Autodesk Inventor part; units mm, degrees
ref_plane "YZ Plane" through (0, 0, 0) normal (1, 0, 0) x (0, 1, 0)
ref_plane "XZ Plane" through (0, 0, 0) normal (0, 1, 0) x (-1, 0, 0)
ref_plane "XY Plane" through (0, 0, 0) normal (0, 0, 1) x (1, 0, 0)
sketch "Sketch1" plane through (0, 0, 0) normal (0, 1, 0) x (-1, 0, 0)
  line L0 (0, 0) -> (-299.72, 0)
  line L1 (-299.72, 0) -> (-299.72, 222.25)
  line L2 (-299.72, 222.25) -> (0, 222.25)
  line L3 (0, 222.25) -> (0, 0)
  dimension "d0" = 299.72
  dimension "d1" = 222.25
extrude "Extrusion1" add sketch "Sketch1" along normal blind 6.35
sketch "Sketch2" plane through (0, 6.35, 0) normal (0, 1, 0) x (1, 0, 0)
  line L0 (0, 0) -> (0, -222.25)
  line L1 (299.72, -222.25) -> (299.72, 0)
  line L2 (0, -222.25) -> (299.72, -222.25)
  line L3 (299.72, -222.25) -> (299.72, 0)
  line L4 (299.72, 0) -> (0, 0)
  line L5 (0, 0) -> (0, -222.25)
  line L6 (296.545, -219.075) -> (3.175, -219.075)
  line L7 (3.175, -219.075) -> (3.175, -3.175)
  line L8 (3.175, -3.175) -> (296.545, -3.175)
  line L9 (296.545, -3.175) -> (296.545, -219.075)
  point P0 (299.72, -222.25)
  dimension "d4" = 3.175
extrude "Extrusion2" add sketch "Sketch2" along normal blind 76.2
sketch "Sketch3" plane through (0, 6.35, 0) normal (0, 1, 0) x (1, 0, 0)
  line L0 (3.175, -219.075) -> (3.175, -3.175) construction
  line L1 (3.175, -3.175) -> (28.575, -3.175) construction
  line L2 (28.575, -3.175) -> (28.575, -28.575) construction
  line L3 (28.575, -28.575) -> (3.175, -28.575) construction
  line L4 (3.175, -28.575) -> (3.175, -3.175) construction
  line L5 (296.545, -3.175) -> (271.145, -3.175) construction
  line L6 (271.145, -3.175) -> (271.145, -28.575) construction
  line L7 (271.145, -28.575) -> (296.545, -28.575) construction
  line L8 (296.545, -28.575) -> (296.545, -3.175) construction
  line L9 (296.545, -219.075) -> (3.175, -219.075) construction
  line L10 (296.545, -219.075) -> (271.145, -219.075) construction
  line L11 (271.145, -219.075) -> (271.145, -193.675) construction
  line L12 (271.145, -193.675) -> (296.545, -193.675) construction
  line L13 (296.545, -193.675) -> (296.545, -219.075) construction
  line L14 (3.175, -219.075) -> (28.575, -219.075) construction
  line L15 (28.575, -219.075) -> (28.575, -193.675) construction
  line L16 (28.575, -193.675) -> (3.175, -193.675) construction
  line L17 (3.175, -193.675) -> (3.175, -219.075) construction
  line L18 (3.175, -193.675) -> (28.575, -219.075) construction
  line L19 (28.575, -193.675) -> (3.175, -219.075) construction
  line L20 (271.145, -193.675) -> (296.545, -219.075) construction
  line L21 (296.545, -219.075) -> (296.545, -193.675) construction
  line L22 (296.545, -193.675) -> (271.145, -219.075) construction
  line L23 (271.145, -3.175) -> (296.545, -28.575) construction
  line L24 (296.545, -3.175) -> (271.145, -28.575) construction
  line L25 (3.175, -3.175) -> (28.575, -28.575) construction
  line L26 (28.575, -3.175) -> (3.175, -28.575) construction
  circle A0 centre (15.875, -15.875) radius 2.3812
  circle A1 centre (283.845, -15.875) radius 2.3812
  circle A2 centre (283.845, -206.375) radius 2.3812
  circle A3 centre (15.875, -206.375) radius 2.3813
  point P0 (0, 0)
  dimension "d7" = 25.4
  dimension "d8" = 25.4
  dimension "d9" = 25.4
  dimension "d10" = 25.4
  dimension "d11" = 25.4
  dimension "d12" = 25.4
  dimension "d13" = 25.4
  dimension "d14" = 25.4
  dimension "d15" = 4.7625
  dimension "d16" = 4.7625
  dimension "d17" = 4.7625
  dimension "d18" = 4.7625
extrude "Extrusion3" cut sketch "Sketch3" against normal blind 6.35
sketch "Sketch4" plane through (3.175, 6.35, 219.075) normal (1, 0, 0) x (0, 0, -1)
  line L0 (215.9, 0) -> (0, 0) construction
  line L1 (0, 0) -> (25.4, 0) construction
  line L2 (25.4, 0) -> (25.4, 25.4) construction
  line L3 (25.4, 25.4) -> (0, 25.4) construction
  line L4 (0, 25.4) -> (0, 0) construction
  line L5 (215.9, 0) -> (190.5, 0) construction
  line L6 (190.5, 0) -> (190.5, 25.4) construction
  line L7 (190.5, 25.4) -> (215.9, 25.4) construction
  line L8 (215.9, 25.4) -> (215.9, 0) construction
  line L9 (0, 25.4) -> (25.4, 0) construction
  line L10 (25.4, 25.4) -> (0, 0) construction
  line L11 (190.5, 25.4) -> (215.9, 0) construction
  line L12 (215.9, 25.4) -> (190.5, 0) construction
  circle A0 centre (203.2, 12.7) radius 2.3813
  circle A1 centre (12.7, 12.7) radius 2.3813
  point P0 (219.075, -6.35)
  dimension "d21" = 25.4
  dimension "d22" = 25.4
  dimension "d23" = 25.4
  dimension "d24" = 25.4
  dimension "d25" = 4.7625
  dimension "d26" = 4.7625
extrude "Extrusion4" cut sketch "Sketch4" against normal blind 3.175
sketch "Sketch5" plane through (3.175, 6.35, 3.175) normal (0, 0, 1) x (1, 0, 0)
  line L0 (0, 0) -> (0, 76.2) construction
  line L1 (0, 0) -> (25.4, 0) construction
  line L2 (25.4, 0) -> (25.4, 25.4) construction
  line L3 (25.4, 25.4) -> (0, 25.4) construction
  line L4 (0, 25.4) -> (0, 0) construction
  line L5 (293.37, 0) -> (267.97, 0) construction
  line L6 (267.97, 0) -> (267.97, 25.4) construction
  line L7 (267.97, 25.4) -> (293.37, 25.4) construction
  line L8 (293.37, 25.4) -> (293.37, 0) construction
  line L9 (0, 25.4) -> (25.4, 0) construction
  line L10 (293.37, 0) -> (0, 0) construction
  line L11 (25.4, 25.4) -> (0, 0) construction
  line L12 (293.37, 25.4) -> (267.97, 0) construction
  line L13 (293.37, 0) -> (293.37, 76.2) construction
  line L14 (267.97, 25.4) -> (293.37, 0) construction
  circle A0 centre (280.67, 12.7) radius 2.3812
  circle A1 centre (12.7, 12.7) radius 2.3813
  point P0 (-3.175, -6.35)
  dimension "d29" = 25.4
  dimension "d30" = 25.4
  dimension "d31" = 25.4
  dimension "d32" = 25.4
  dimension "d33" = 4.7625
  dimension "d34" = 4.7625
extrude "Extrusion5" cut sketch "Sketch5" against normal blind 3.175
sketch "Sketch6" plane through (296.545, 6.35, 3.175) normal (-1, 0, 0) x (0, 0, 1)
  line L0 (215.9, 0) -> (0, 0) construction
  line L1 (0, 0) -> (25.4, 0) construction
  line L2 (25.4, 0) -> (25.4, 25.4) construction
  line L3 (25.4, 25.4) -> (0, 25.4) construction
  line L4 (0, 25.4) -> (0, 0) construction
  line L5 (215.9, 0) -> (190.5, 0) construction
  line L6 (190.5, 0) -> (190.5, 25.4) construction
  line L7 (190.5, 25.4) -> (215.9, 25.4) construction
  line L8 (215.9, 25.4) -> (215.9, 0) construction
  line L9 (190.5, 0) -> (215.9, 25.4) construction
  line L10 (215.9, 0) -> (215.9, 76.2) construction
  line L11 (190.5, 25.4) -> (215.9, 0) construction
  line L12 (0, 25.4) -> (25.4, 0) construction
  line L13 (25.4, 25.4) -> (0, 0) construction
  circle A0 centre (12.7, 12.7) radius 2.3812
  circle A1 centre (203.2, 12.7) radius 2.3813
  point P0 (-3.175, -6.35)
  dimension "d37" = 25.4
  dimension "d38" = 25.4
  dimension "d39" = 25.4
  dimension "d40" = 25.4
  dimension "d41" = 4.7625
  dimension "d42" = 4.7625
extrude "Extrusion6" cut sketch "Sketch6" against normal blind 3.175
sketch "Sketch7" plane through (296.545, 6.35, 219.075) normal (0, 0, -1) x (-1, 0, 0)
  line L0 (293.37, 0) -> (267.97, 0) construction
  line L1 (267.97, 0) -> (267.97, 25.4) construction
  line L2 (267.97, 25.4) -> (293.37, 25.4) construction
  line L3 (293.37, 25.4) -> (293.37, 0) construction
  line L4 (293.37, 0) -> (0, 0) construction
  line L5 (0, 0) -> (25.4, 0) construction
  line L6 (25.4, 0) -> (25.4, 25.4) construction
  line L7 (25.4, 25.4) -> (0, 25.4) construction
  line L8 (0, 25.4) -> (0, 0) construction
  line L9 (0, 25.4) -> (25.4, 0) construction
  line L10 (25.4, 25.4) -> (0, 0) construction
  line L11 (267.97, 0) -> (293.37, 25.4) construction
  line L12 (267.97, 25.4) -> (293.37, 0) construction
  circle A0 centre (280.67, 12.7) radius 2.3812
  circle A1 centre (12.7, 12.7) radius 2.3813
  point P0 (296.545, -6.35)
  dimension "d45" = 25.4
  dimension "d46" = 25.4
  dimension "d47" = 25.4
  dimension "d48" = 25.4
  dimension "d49" = 4.7625
  dimension "d50" = 4.7625
extrude "Extrusion7" cut sketch "Sketch7" against normal blind 3.175
sketch "Sketch8" plane through (3.175, 6.35, 219.075) normal (1, 0, 0) x (0, 0, -1)
  line L0 (215.9, 0) -> (0, 0) construction
  line L1 (0, 0) -> (107.95, 0) construction
  line L2 (107.95, 0) -> (130.175, 0) construction
  line L3 (107.95, 0) -> (130.175, 0) construction
  line L4 (130.175, 0) -> (85.725, 0) construction
  line L5 (85.725, 0) -> (85.725, 20.6375) construction
  line L6 (85.725, 20.6375) -> (130.175, 20.6375) construction
  line L7 (130.175, 20.6375) -> (130.175, 0) construction
  line L8 (85.725, 0) -> (85.725, 10.3251) construction
  line L9 (130.175, 0) -> (130.175, 10.3251) construction
  line L10 (130.175, 0) -> (140.5001, 0) construction
  line L11 (85.725, 10.3251) -> (87.3125, 10.3251) construction
  line L12 (130.175, 10.3251) -> (128.5875, 10.3251) construction
  line L13 (128.5875, 10.3251) -> (120.65, 10.3251) construction
  line L14 (128.5875, 10.3251) -> (136.525, 10.3251) construction
  line L15 (87.3125, 10.3251) -> (95.25, 10.3251) construction
  line L16 (87.3125, 10.3251) -> (95.25, 10.3251) construction
  circle A0 centre (95.25, 10.3251) radius 7.9375
  circle A1 centre (120.65, 10.3251) radius 7.9375
  dimension "d53" = 107.95
  dimension "d54" = 22.225
  dimension "d55" = 0
  dimension "d56" = 44.45
  dimension "d57" = 20.6375
  dimension "d58" = 10.3251
  dimension "d59" = 10.3251
  dimension "d60" = 90
  dimension "d61" = 1.5875
  dimension "d62" = 1.5875
  dimension "d64" = 7.9375
  dimension "d65" = 180
  dimension "d66" = 7.9375
  dimension "d67" = 0
  dimension "d68" = 15.875
  dimension "d69" = 15.875
extrude "Extrusion8" cut sketch "Sketch8" against normal blind 3.175
properties part number "Lower Chassis_2"
Input: part model. Units: mm. Frame: model coordinates. A direction names the side the tool comes from. Coordinates: 2 decimals unless noted, no trailing zeros. Loops run counter-clockwise (first coordinate to the right, second up) from the corner with the lowest first, then second, coordinate; pieces in that order, holes last. Notation, with made-up numbers: (69, 61) -> (88, 61) arc R15 cw to (88, 67) -> close; hole circle Ø10 at (-20, -15.5). An arc over 180 degrees is marked (long way). Write item = value, one per line. Start each with the question number.
Item 1: Cut plane B-B, the plane x = 162. Return loops of the section in (y, z) (3 decimals).
Item 2: Material intervals for line 1 (Z direction, x = 279.5, y = 38) (3 decimals); line 2 (X direction, y = 52, z = 30.5) (3 decimals); line 3 (Z direction, x = 2, y = 19), sorted ascending.
Item 3: First-contact query: P1, Ø4, axis at x = 15.875, z = 15.875, coming from the -Y side; P2, Ø7.5, axis at x = 283.845, z = 15.875, coming from the +Y side. Flat tips, straight axial feed; report the tip coordinate or a pass-through.
Item 4: Cut plane A-A, the plane y = 67. Return loops of the section in (x, z) (3 decimals), plus the area to 3 significant figures.
Item 5: Reachability of faces 5 (the face through (299.72, 41, 110)), 6 (the face through (152, 44, 219.075)), 7 (the face through (1.61, 13.635, 116.493)) from +Z, -Z, +X, -X, +Y, -Y: full face, straight path, thin tool, end or side. Return the list, or none.
Item 6: Cut plane C-C, the plane z = 148. Return loops of the section in (x, y) (3 decimals), plus the area to 3 significant figures.
Item 7: Mould query, pull axis Z, two halves, no side actions, for faces 1 (the face through (148, 44, 3.175)), 2 (the face through (1.61, 13.635, 91.093)), 3 (the face through (152, 41, 222.25)), 4 (the face through (0, 41, 113)). Classes: pulls with the +Z half, pulls with the -Z half, needs draft (parallel to the pull), parting line crosses it, or undercut.
Ans:
q1.outline = (0, 0) -> (82.55, 0) -> (82.55, 3.175) -> (6.35, 3.175) -> (6.35, 219.075) -> (82.55, 219.075) -> (82.55, 222.25) -> (0, 222.25) -> close
q2.line_1 = 0 to 3.175, 219.075 to 222.25
q2.line_2 = 0 to 3.175, 296.545 to 299.72
q2.line_3 = 0 to 13.49, 18.26 to 90.84, 106.01 to 116.24, 131.41 to 203.99, 208.76 to 222.25
q3.P1 = through
q3.P2 = 6.35
q4.outline = (0, 0) -> (299.72, 0) -> (299.72, 222.25) -> (0, 222.25) -> close; hole (3.175, 3.175) -> (296.545, 3.175) -> (296.545, 219.075) -> (3.175, 219.075) -> close
q4.area = 3,270 mm²
q5.face_5 = +Z, -Z, +X, +Y, -Y
q5.face_6 = +Y
q5.face_7 = -X
q6.outline = (0, 0) -> (299.72, 0) -> (299.72, 82.55) -> (296.545, 82.55) -> (296.545, 6.35) -> (3.175, 6.35) -> (3.175, 82.55) -> (0, 82.55) -> close
q6.area = 2,390 mm²
q7.face_1 = undercut
q7.face_2 = undercut
q7.face_3 = pulls with the +Z half
q7.face_4 = needs draft
